Part model, mm, in its own coordinate system. Face numbers are marked on the shaded views. A direction names the side the tool comes from. Round coordinates to 2 decimals unless told otherwise and drop trailing zeros. Write each loop counter-clockwise with the first axis right and the second up, starting at its lowest first coordinate (ties: lowest second). Pieces come first, ordered by that corner, then holes. Notation, with made-up numbers: M -39,37.25 L -2,37.25 A32 cw -2,66.25 Z; hole C -32.75,47.25 d10. An arc over 180 degrees is marked long. One line per question, with ' | ' between items. Start each with the question number.
1) Saw through at A-A (x = 0). List the corners of the cut face in (y, z).
2) Drop flat-ended pins along their axis: pin 1 Ø1.5 at (y, z) = (-3.5, 2) entering from +X; pin 2 Ø1.5 at (x, z) = (19.5, 3) entering from -Y; pin 3 Ø2 at (y, z) = (3, -3.5) entering from +X. Give the stop position or say it passes through.
3) Saw through at B-B (y = -2.5). List the corners of the cut face in (x, z).
4) Mould opens along X. For the marked faces 1, 2, 3 and 4 say: pulls with the +X half, pulls with the -X half, needs draft (parallel to the pull), parting line crosses it, or undercut.
5) Saw through at C-C (z = 2). List the corners of the cut face in (x, y), plus the area to 3 significant figures.
6) Wall check: probe 1 along Y at (x, z) = (0, -4.25); probe 2 along X at (y, z) = (20, -11); probe 3 along Z at (x, y) = (-4, 18.5). Give the ranges that are in metal, low to high. Write a range as [from, to].
7) Saw through at D-D (x = -10). List the corners of the cut face in (y, z), plus the area to 3 significant figures.
8) Tool access for the marked faces 5, 6 and 7: list every direction of +Z, -Z, +X, -X, +Y, -Y with a clear straight run to the whole face (end or side of a thin tool).
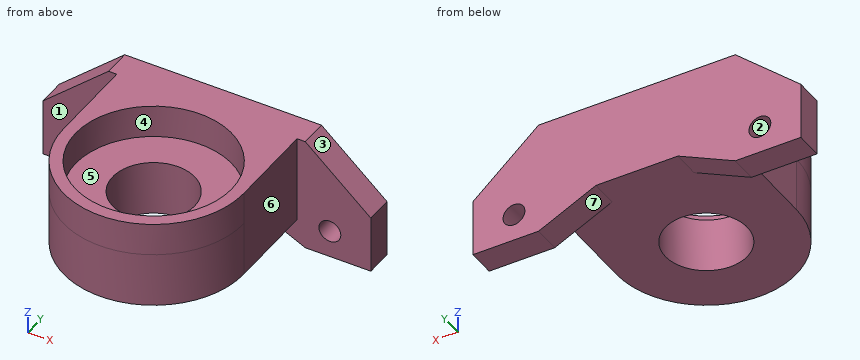
```python
from build123d import *

# Parameters (mm, degrees)
ESQUISSE1_R             = 16.5
ESQUISSE1_R_2           = 14.29
BOSS_EXTRU_1_DEPTH      = 6
BOSS_EXTRU_2_START      = 10
ESQUISSE2_R             = 16.5
BOSS_EXTRU_2_DEPTH      = 10
BOSS_EXTRU_3_DEPTH      = 5
BOSS_EXTRU_4_DEPTH      = 16
ESQUISSE7_R             = 2
ESQUISSE7_W             = 60
ESQUISSE7_H             = 4
ENL_V_MAT_EXTRU_1_DEPTH = 57.071383076
ESQUISSE8_R             = 7.5
ENL_V_MAT_EXTRU_2_DEPTH = 39.23937761
ESQUISSE10_W            = 60
ESQUISSE10_H            = 5
BOSS_EXTRU_5_DEPTH      = 5
ESQUISSE11_W            = 15
ESQUISSE11_H            = 5
ENL_V_MAT_EXTRU_4_DEPTH = 5


with BuildPart() as part:
    # Esquisse1 → Boss.-Extru.1 (new body)
    with BuildSketch(Plane.XY):
        Circle(ESQUISSE1_R)
        Circle(ESQUISSE1_R_2, mode=Mode.SUBTRACT)
    extrude(amount=BOSS_EXTRU_1_DEPTH)

    # Esquisse2 → Boss.-Extru.2 (add)
    with BuildSketch(Plane(origin=(0, 0, 0), x_dir=(-1, 0, 0), z_dir=(0, 0, -1)).offset(BOSS_EXTRU_2_START)):
        Circle(ESQUISSE2_R)
    extrude(amount=-BOSS_EXTRU_2_DEPTH)



with BuildPart() as body_2:
    # Esquisse3 → Boss.-Extru.3 (new body)
    with BuildSketch(Plane(origin=(0, 16.5, 0), x_dir=(1, 0, 0), z_dir=(0, 1, 0))):
        Polygon((0, 10), (40, 10), (40, -10), (0, -10), (-40, -10), (-40, 10), align=None)
    extrude(amount=BOSS_EXTRU_3_DEPTH)


with BuildPart() as part_1:
    add(part.part)

    add(body_2.part)  # Boss.-Extru.4 merges body 2
    # Esquisse4 → Boss.-Extru.4 (add)
    with BuildSketch(Plane.XY.offset(-10)):
        with BuildLine():
            ThreePointArc((-16.5, 0), (-11.66726189, 11.66726189), (0, 16.5))
            Line((0, 16.5), (-16.5, 16.5))
            Line((-16.5, 16.5), (-16.5, 0))
        make_face()
        with BuildLine():
            ThreePointArc((16.5, 0), (11.66726189, 11.66726189), (0, 16.5))
            Line((0, 16.5), (16.5, 16.5))
            Line((16.5, 16.5), (16.5, 0))
        make_face()
    extrude(amount=BOSS_EXTRU_4_DEPTH)

    # Esquisse7 → Enlèv. mat.-Extru.1 (cut, through all)
    with BuildSketch(Plane(origin=(0, 21.5, 0), x_dir=(1, 0, 0), z_dir=(0, 1, 0))):
        Polygon((-40, -10), (-30, -10), (-30, -6), (-30, 10), (-40, 10), align=None)
        Polygon((30, -6), (30, -10), (40, -10), (40, 10), (30, 10), align=None)
        with Locations((22.5, 10)):
            Circle(ESQUISSE7_R)
        with Locations((-22.5, 10)):
            Circle(ESQUISSE7_R)
        with Locations((0, -8)):
            Rectangle(ESQUISSE7_W, ESQUISSE7_H)
    extrude(amount=-ENL_V_MAT_EXTRU_1_DEPTH, mode=Mode.SUBTRACT)

    # Esquisse8 → Enlèv. mat.-Extru.2 (cut, through all)
    with BuildSketch(Plane.XY):
        Circle(ESQUISSE8_R)
    extrude(amount=-ENL_V_MAT_EXTRU_2_DEPTH, mode=Mode.SUBTRACT)

    # Esquisse10 → Boss.-Extru.5 (add)
    with BuildSketch(Plane(origin=(0, 0, -10), x_dir=(-1, 0, 0), z_dir=(0, 0, -1))):
        with Locations((0, 19)):
            Rectangle(ESQUISSE10_W, ESQUISSE10_H)
    extrude(amount=BOSS_EXTRU_5_DEPTH)

    # Esquisse11 → Enlèv. mat.-Extru.4 (cut)
    with BuildSketch(Plane(origin=(0, 21.5, 0), x_dir=(1, 0, 0), z_dir=(0, 1, 0))):
        Polygon((-18, -6), (-30, 4.5), (-30, -6), align=None)
        Polygon((30, 4.5), (18, -6), (30, -6), align=None)
        with BuildLine():
            Line((20.5, 10), (24.5, 10))
            ThreePointArc((24.5, 10), (22.5, 12), (20.5, 10))
        make_face()
        with BuildLine():
            ThreePointArc((20.5, 10), (22.5, 8), (24.5, 10))
            Line((24.5, 10), (20.5, 10))
        make_face()
        with BuildLine():
            Line((-24.5, 10), (-20.5, 10))
            ThreePointArc((-20.5, 10), (-22.5, 12), (-24.5, 10))
        make_face()
        with BuildLine():
            ThreePointArc((-24.5, 10), (-22.5, 8), (-20.5, 10))
            Line((-20.5, 10), (-24.5, 10))
        make_face()
        Polygon((-7.5, 15), (-18, 15), (-7.5, 10), align=None)
        with Locations((0, 12.5)):
            Rectangle(ESQUISSE11_W, ESQUISSE11_H)
        Polygon((7.5, 10), (18, 15), (7.5, 15), align=None)
    extrude(amount=-ENL_V_MAT_EXTRU_4_DEPTH, mode=Mode.SUBTRACT)


solid = part_1.part
```
Answer key:
1) outline: M -16.5,-10 L -7.5,-10 L -7.5,0 L -14.29,0 L -14.29,6 L -16.5,6 Z; M 7.5,-10 L 21.5,-10 L 21.5,6 L 14.29,6 L 14.29,0 L 7.5,0 Z
2) pin 1: stops at x = 16.27 | pin 2: stops at y = 16.5 | pin 3: stops at x = 16.5
3) outline: M -16.31,-10 L -7.07,-10 L -7.07,0 L -14.07,0 L -14.07,6 L -16.31,6 Z; M 7.07,-10 L 16.31,-10 L 16.31,6 L 14.07,6 L 14.07,0 L 7.07,0 Z
4) face 1: needs draft | face 2: undercut | face 3: pulls with the +X half | face 4: undercut
5) outline: M -22.57,16.5 L -16.5,16.5 L -16.5,0 A16.5 ccw 16.5,0 L 16.5,16.5 L 22.57,16.5 L 22.57,21.5 L -22.57,21.5 Z; hole C 0,0 d28.58 | area: 556 mm2
6) probe 1: y = [-16.5, -7.5], [7.5, 21.5] | probe 2: x = [-30, -24.23], [-20.77, -9.6], [9.6, 20.77], [24.23, 30] | probe 3: z = [-10, 6]
7) outline: M -13.12,-10 L 16.5,-10 L 16.5,-11.19 L 21.5,-11.19 L 21.5,6 L 10.21,6 L 10.21,0 L -10.21,0 L -10.21,6 L -13.12,6 Z | area: 437 mm2
8) face 5: +Z | face 6: +Z, -Z, +X, -Y | face 7: -Z, +Y, -Y
